Verification items for the finished model (mm, model axes). Give positions to 0.01 mm unless a question says otherwise; leave off trailing zeros. Loops run counter-clockwise (first coordinate to the right, second up) from the corner with the lowest first, then second, coordinate; pieces in that order, holes last. Notation, with made-up numbers: (1.25, 45.25) - (11.25, 45.25) arc R26 ccw to (11.25, 66.25) - close; hole circle Ø6 at (-28, 24.25). An arc over 180 degrees is marked (long way). Put each result on its own line as item: value. Start each with the question number.
```python
from build123d import *

# Parameters (mm, degrees)
SKETCH_1_W          = 76.2
SKETCH_1_H          = 30
EXTRUDE_1_DEPTH     = 3
SKETCH_2_W          = 19.6215
SKETCH_2_H          = 3
CUT_EXTRUDE_1_DEPTH = 3
SKETCH_3_W          = 3
SKETCH_3_H          = 8.89
CUT_EXTRUDE_2_DEPTH = 3
SKETCH_4_W          = 30.7975
SKETCH_4_H          = 3
EXTRUDE_2_DEPTH     = 3
SKETCH_6_R          = 10.16
SKETCH_6_R_2        = 7.62
CUT_EXTRUDE_4_DEPTH = 3


with BuildPart() as part:
    # 스케치1 → 보스-돌출1 (new body)
    with BuildSketch(Plane.XY):
        Rectangle(SKETCH_1_W, SKETCH_1_H)
    extrude(amount=EXTRUDE_1_DEPTH)

    # 스케치2 → 컷-돌출1 (cut)
    with BuildSketch(Plane.XY.offset(3)):
        with Locations((-28.28925, -13.5)):
            Rectangle(SKETCH_2_W, SKETCH_2_H)
        with Locations((28.28925, -13.5)):
            Rectangle(SKETCH_2_W, SKETCH_2_H)
    extrude(amount=-CUT_EXTRUDE_1_DEPTH, mode=Mode.SUBTRACT)

    # 스케치3 → 컷-돌출2 (cut)
    with BuildSketch(Plane.XY.offset(3)):
        with Locations((-36.6, 1.5)):
            Rectangle(SKETCH_3_W, SKETCH_3_H)
        with Locations((36.6, 1.5)):
            Rectangle(SKETCH_3_W, SKETCH_3_H)
    extrude(amount=-CUT_EXTRUDE_2_DEPTH, mode=Mode.SUBTRACT)

    # 스케치4 → 보스-돌출2 (add)
    with BuildSketch(Plane.XY.offset(3)):
        with Locations((0, 16.5)):
            Rectangle(SKETCH_4_W, SKETCH_4_H)
    extrude(amount=-EXTRUDE_2_DEPTH)

    # 스케치6 → 컷-돌출4 (cut)
    with BuildSketch(Plane.XY.offset(3)):
        with Locations((0, 1.5)):
            Circle(SKETCH_6_R)
        with Locations((-22.86, 1.5)):
            Circle(SKETCH_6_R_2)
        with Locations((22.86, 1.5)):
            Circle(SKETCH_6_R_2)
    extrude(amount=-CUT_EXTRUDE_4_DEPTH, mode=Mode.SUBTRACT)


solid = part.part
```
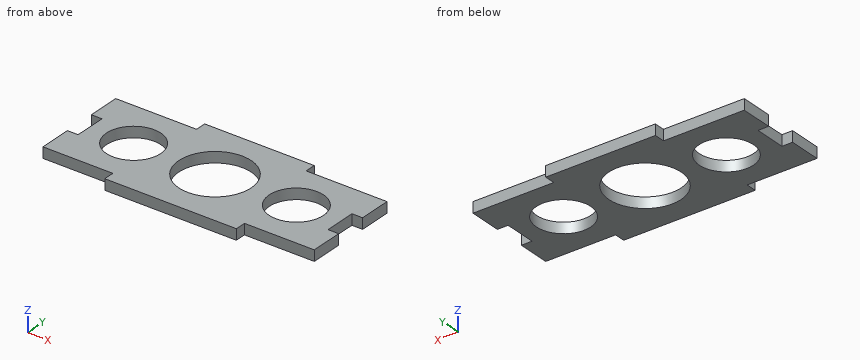
1) Section check C-C, the plane z = 0.95. Enter the section's corners in (x, y) (1 decimal), plus the area to 3 significant figures.
2) Section check B-B, the plane y = 1.5. Enter the section's corners in (x, z).
3) Section check D-D, the plane y = -7. Enter the section's corners in (x, z).
4) Section check A-A, the plane x = 22.86. Enter the section's corners in (y, z), plus the area to 3 significant figures.
5) Scan lines: line 1 along Y through (x, z) = (-22.86, 1.75); line 2 along Y through (x, z) = (0, 1.2); line 3 along Y through (x, z) = (32, 1.9). Record each from-to range of solid material in increasing order. Write a range as from..to.
6) Depth check by flat-ended pin: P1, Ø1.5, axis at y = 3, z = 1.5, coming from the +X side; P2, Ø1.5, axis at x = -36.5, z = 2, coming from the -Y side; P3, Ø0.9, axis at y = -13.5, z = 1, coming from the -X side. Enter the tip coordinate at first touch or a pass-through.
Results are:
1. outline: (-38.1, -12) - (-18.5, -12) - (-18.5, -15) - (18.5, -15) - (18.5, -12) - (38.1, -12) - (38.1, -2.9) - (35.1, -2.9) - (35.1, 5.9) - (38.1, 5.9) - (38.1, 15) - (15.4, 15) - (15.4, 18) - (-15.4, 18) - (-15.4, 15) - (-38.1, 15) - (-38.1, 5.9) - (-35.1, 5.9) - (-35.1, -2.9) - (-38.1, -2.9) - close; hole circle Ø15.2 at (-22.9, 1.5); hole circle Ø20.3 at (0, 1.5); hole circle Ø15.2 at (22.9, 1.5)
1. area: 1,520 mm2
2. outline: (-35.1, 0) - (-30.48, 0) - (-30.48, 3) - (-35.1, 3) - close; (-15.24, 0) - (-10.16, 0) - (-10.16, 3) - (-15.24, 3) - close; (10.16, 0) - (15.24, 0) - (15.24, 3) - (10.16, 3) - close; (30.48, 0) - (35.1, 0) - (35.1, 3) - (30.48, 3) - close
3. outline: (-38.1, 0) - (-5.57, 0) - (-5.57, 3) - (-38.1, 3) - close; (5.57, 0) - (38.1, 0) - (38.1, 3) - (5.57, 3) - close
4. outline: (-12, 0) - (-6.12, 0) - (-6.12, 3) - (-12, 3) - close; (9.12, 0) - (15, 0) - (15, 3) - (9.12, 3) - close
4. area: 35.3 mm2
5. line 1: y = -12..-6.12, 9.12..15
5. line 2: y = -15..-8.66, 11.66..18
5. line 3: y = -12..15
6. P1: stops at x = 35.1
6. P2: stops at y = -12
6. P3: stops at x = -18.48
